Geometry: final body of the model. Coordinates: model frame, mm. Face numbers are marked on the shaded views. Give positions to 0.01 mm unless a question says otherwise; leave off trailing zeros. Order: outer loops, then holes, each group sorted by start corner. A loop starts at its lowest first (then second) coordinate and runs counter-clockwise, first axis right, second up. Notation, with made-up numbers: (45.5, 78.5) -> (73.5, 78.5) arc R35 cw to (73.5, 112.5) -> close; hole circle Ø11 at (-5.75, 50.5). An arc over 180 degrees is marked (long way). One line per question, with ' | ' between items.
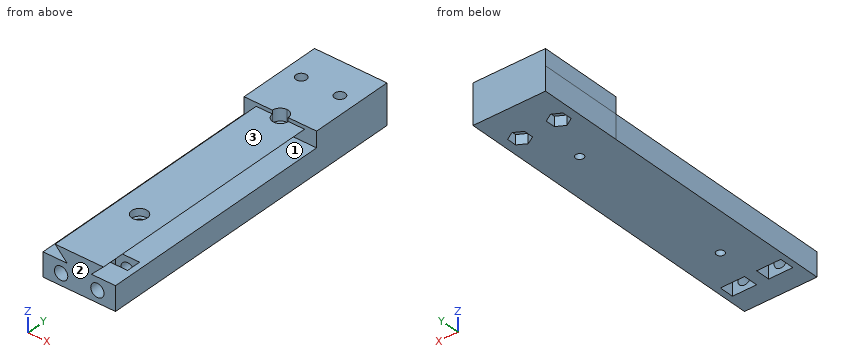
from build123d import *

# Parameters (mm, degrees)
F0_R            = 2.5000000706
F0_R_2          = 2.5000000298
F1_DEPTH        = 100
F3_DEPTH        = 35
F6_D            = 4.4
F6_DEPTH        = 40
F6_TIP          = 1.3218933619
F5_W            = 10
F5_H            = 6
F7_DEPTH        = 10
F9_D            = 5.5
F9_DEPTH        = 40
F9_TIP          = 1.6523667023
F10_DEPTH       = 4
F12_D           = 3.3
F12_CBORE_D     = 6.5
F12_CBORE_DEPTH = 3
F14_DEPTH       = 5


# Not quite as in the source:
# - ends of sketch curves that miss each other by under 0.0002 mm in the source are joined
# - a feature names something its author has since deleted; it is built from what else it names


with BuildPart() as f1:
    # F0 (on Front) → F1 (new body)
    with BuildSketch(Plane.XZ):
        Polygon((-39.8704047501, 4.2457092745), (-39.8704047501, -5.5542903855), (-9.8704054207, -5.5542903855), (-9.8704054207, 4.4457092745), (-19.8704054207, 4.4457092745), (-14.8704054207, 9.4457092745), (-24.8704050854, 9.4457092745), (-34.8704047501, 9.4457092745), (-29.8704047501, 4.2457092745), align=None)
        with Locations((-32.3704050442, -0.7542907016)):
            Circle(F0_R, mode=Mode.SUBTRACT)
        with Locations((-17.3704050202, -0.7062930843)):
            Circle(F0_R_2, mode=Mode.SUBTRACT)
        with Locations((-32.3704050442, -0.7542907016)):
            Circle(F0_R)
        with Locations((-17.3704050202, -0.7062930843)):
            Circle(F0_R_2)
    extrude(amount=F1_DEPTH)

    # F2 (on face) → F3 (join)
    with BuildSketch(Plane(origin=(0, 0, 0), x_dir=(-1, 0, 0), z_dir=(0, 1, 0))):
        Polygon((9.8704054207, 4.4457092745), (9.8704054207, -5.5542903855), (39.8704054207, -5.5542903855), (39.8704054207, 4.2457092745), (29.8704047501, 4.2457092745), (34.8704047501, 9.4457092745), (14.8704054207, 9.4457092745), (19.8704054207, 4.4457092745), align=None)
        Polygon((9.8704054207, 10.9457096145), (9.8704054207, 4.4457092745), (19.8704054207, 4.4457092745), (14.8704054207, 9.4457092745), (34.8704047501, 9.4457092745), (29.8704047501, 4.2457092745), (39.8704047501, 4.2457092745), (39.8704054207, 10.9457096145), align=None)
    extrude(amount=F3_DEPTH)

    # F4: union 

    # F6
    with Locations(Plane(origin=(0, 0, -5.5542903855), x_dir=(1, 0, 0), z_dir=(0, 0, -1))):
        with Locations((-16.8704054207, -20), (-32.8704047501, -20)):
            Hole(F6_D / 2, depth=F6_DEPTH)
            with Locations((0, 0, -(F6_DEPTH + F6_TIP / 2))):  # 118° drill point
                Cone(0, F6_D / 2, F6_TIP, mode=Mode.SUBTRACT)

    # F5 (on face) → F7 (cut)
    with BuildSketch(Plane(origin=(0, 0, -5.5542903855), x_dir=(1, 0, 0), z_dir=(0, 0, -1))):
        with Locations((-17.3704054207, 88)):
            Rectangle(F5_W, F5_H)
        with Locations((-32.3704047501, 88)):
            Rectangle(F5_W, F5_H)
    extrude(amount=-F7_DEPTH, mode=Mode.SUBTRACT)

    # F9
    with Locations(Plane.XZ.offset(100)):
        with Locations((-32.3704050442, -0.7542907016), (-17.3704050202, -0.7062930843)):
            Hole(F9_D / 2, depth=F9_DEPTH)
            with Locations((0, 0, -(F9_DEPTH + F9_TIP / 2))):  # 118° drill point
                Cone(0, F9_D / 2, F9_TIP, mode=Mode.SUBTRACT)

    # F5 (on face) → F10 (cut)
    with BuildSketch(Plane(origin=(0, 0, -5.5542903855), x_dir=(1, 0, 0), z_dir=(0, 0, -1))):
        Polygon((-20.3704054207, -17.9792740578), (-20.3704054207, -22.0207259422), (-16.8704054207, -24.0414518843), (-13.3704054207, -22.0207259422), (-13.3704054207, -17.9792740578), (-16.8704054207, -15.9585481157), align=None)
        Polygon((-32.7971248335, -24.0407874712), (-29.3343401905, -21.9569314662), (-29.4076201071, -17.9161439951), (-32.9436846667, -15.9592125288), (-36.4064693097, -18.0430685338), (-36.3331893931, -22.0838560049), align=None)
    extrude(amount=-F10_DEPTH, mode=Mode.SUBTRACT)

    # F12 (through all)
    with Locations(Plane.XY.offset(9.4457092745)):
        with Locations((-24.8704050854, 0), (-24.8704050854, -70)):
            CounterBoreHole(F12_D / 2, F12_CBORE_D / 2, F12_CBORE_DEPTH)

    # F13 (on face) → F14 (cut)
    with BuildSketch(Plane.XY.offset(10.9457096145)):
        with BuildLine():
            Line((-28.1204054207, 0), (-21.6204054207, 0))
            ThreePointArc((-21.6204054207, 0), (-24.8704054207, 3.25), (-28.1204054207, 0))
        make_face()
    extrude(amount=-F14_DEPTH, mode=Mode.SUBTRACT)


solid = f1.part
1) Section C-C on y = 20. Return loops of the section in (x, z), plus the area to 3 significant figures.
Check result:
outline: (-39.87, -5.55) -> (-36.37, -5.55) -> (-36.37, -1.55) -> (-35.07, -1.55) -> (-35.07, 10.95) -> (-39.87, 10.95) -> (-39.87, 4.25) -> close; (-30.67, -1.55) -> (-29.37, -1.55) -> (-29.37, -5.55) -> (-20.37, -5.55) -> (-20.37, -1.55) -> (-19.07, -1.55) -> (-19.07, 10.95) -> (-30.67, 10.95) -> close; (-14.67, -1.55) -> (-13.37, -1.55) -> (-13.37, -5.55) -> (-9.87, -5.55) -> (-9.87, 10.95) -> (-14.67, 10.95) -> close | area: 329 mm^2
2) Pull-direction query (Z, two-part tool) for the marked faces 1, 2 and 3; classes: +Z half, -Z half, draft (parallel to the pull), parting line (faces both ways), or undercut.
Check result:
face 1: undercut | face 2: draft | face 3: +Z half
3) Section B-B on y = -70. Return loops of the section in (x, z), plus the area to 3 significant figures.
Check result:
outline: (-39.87, -5.55) -> (-26.52, -5.55) -> (-26.52, 6.45) -> (-28.12, 6.45) -> (-28.12, 9.45) -> (-34.87, 9.45) -> (-29.87, 4.25) -> (-39.87, 4.25) -> close; (-23.22, -5.55) -> (-9.87, -5.55) -> (-9.87, 4.45) -> (-19.87, 4.45) -> (-14.87, 9.45) -> (-21.62, 9.45) -> (-21.62, 6.45) -> (-23.22, 6.45) -> close; hole circle Ø5.5 at (-32.37, -0.75); hole circle Ø5.5 at (-17.37, -0.71) | area: 267 mm^2
4) Contact query for flat-ended pins moving along their axis: pin 1 Ø5.5 at (x, y) = (-17.5, 22) entering from -Z; pin 2 Ø2 at (x, y) = (-36.5, -14) entering from +Z; pin 3 Ø5 at (x, z) = (-32.37, -0.75) entering from -Y; pin 4 Ø4.5 at (x, z) = (-17.37, -0.71) entering from -Y. Output: stop coordinate, or through.
Check result:
pin 1: stops at z = -5.55 | pin 2: stops at z = 4.25 | pin 3: stops at y = -59.85 | pin 4: stops at y = -59.7
5) Material intervals for probe 1 along X at (y, z) = (20, 8.75); probe 2 along Y at (x, z) = (-25, 4.5); probe 3 along Y at (x, z) = (-37, -1), sorted ascending. Write a range as from..to.
Check result:
probe 1: x = -39.87..-35.07, -30.67..-19.07, -14.67..-9.87 | probe 2: y = -100..-71.64, -68.36..-1.64, 1.64..35 | probe 3: y = -100..-91, -85..35
6) Section A-A on y = -89. Return loops of the section in (x, z), plus the area to 3 significant figures.
Check result:
outline: (-39.87, -5.55) -> (-37.37, -5.55) -> (-37.37, 4.25) -> (-39.87, 4.25) -> close; (-34.87, 9.45) -> (-30.06, 4.45) -> (-27.37, 4.45) -> (-27.37, -5.55) -> (-22.37, -5.55) -> (-22.37, 4.45) -> (-19.87, 4.45) -> (-14.87, 9.45) -> close; (-12.37, -5.55) -> (-9.87, -5.55) -> (-9.87, 4.45) -> (-12.37, 4.45) -> close | area: 175 mm^2
